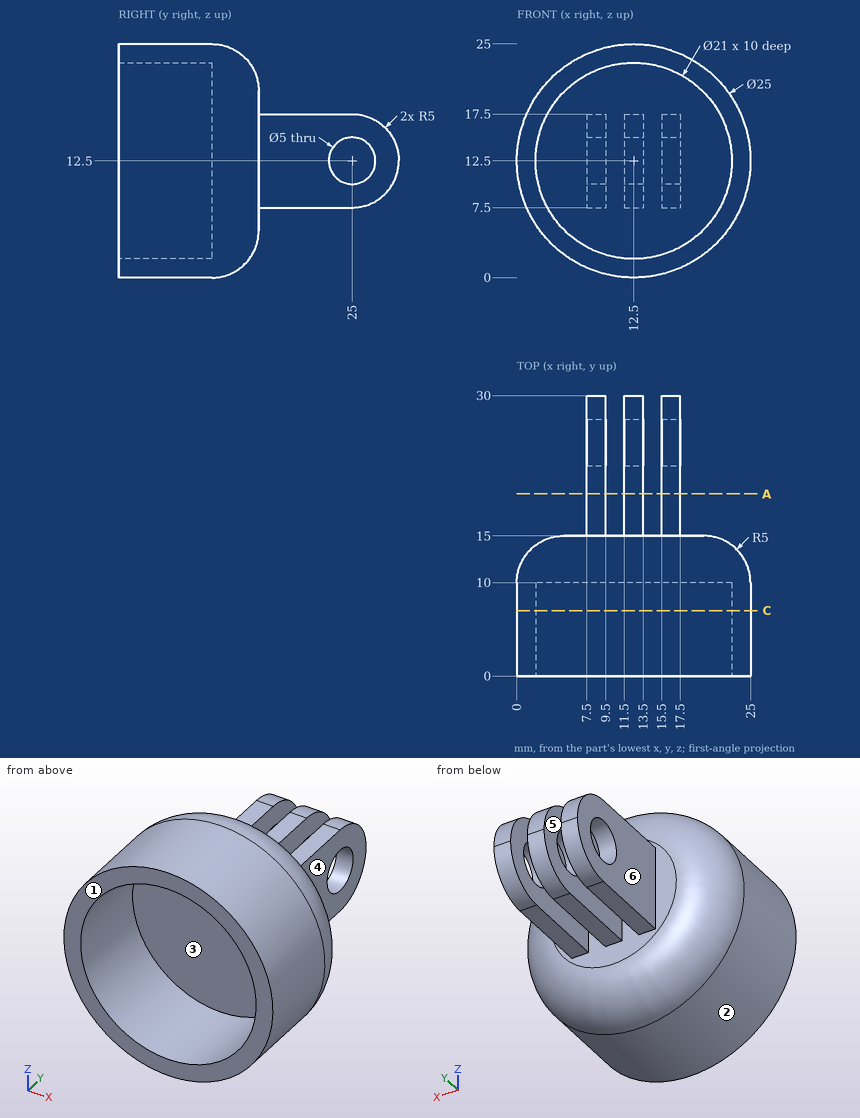
For this review, use the dimensioned drawing (mm, ordinates from the lowest corner) and the shaded views. A direction names the side the tool comes from. Round coordinates to 2 decimals unless told otherwise and drop trailing zeros. Order: outer loops, then holes, each group sorted by start corner. A loop starts at its lowest first (then second) coordinate and runs counter-clockwise, first axis right, second up.
1) Machinability: for the marked faces 4, 5 and 6, which of the approach directions +Z, -Z, +X, -X, +Y, -Y give a long, thin tool a straight path to every point of the face, cutting with its end or side? Answer none if there is none.
The answers:
face 4: +Z, -Z, +X, +Y
face 5: +Z, -Z, +Y
face 6: +Z, -Z, -X, +Y
2) For L1, parallel to Y at x = 12.9, z = 12.5; L2, parallel to X at y = 17, z = 14; L3, parallel to X at y = 7.75, z = 12.5, list the stretches that pass through material, from the lowest coordinate up.
The answers:
L1: y = 10 to 22.5, 27.5 to 30
L2: x = 7.5 to 9.5, 11.5 to 13.5, 15.5 to 17.5
L3: x = 0 to 2, 23 to 25
3) Clearance check with flat-ended pins moving along their axes: pin 1 Ø2 at (x, y) = (13, 18) entering from -Z; pin 2 Ø3 at (x, y) = (16, 12) entering from -Z; pin 3 Ø3 at (y, z) = (22, 12.5) entering from -X; pin 4 Ø12 at (x, z) = (18.5, 4) entering from -Y. State where each tip first meets the part, or that it passes through.
The answers:
pin 1: stops at z = 7.5
pin 2: stops at z = 0.33
pin 3: stops at x = 7.5
pin 4: stops at y = 0
4) Consider section A-A (y = 19.5). State the section outline as (x, z) points.
The answers:
outline: (7.5, 7.5) - (9.5, 7.5) - (9.5, 17.5) - (7.5, 17.5) - close; (11.5, 7.5) - (13.5, 7.5) - (13.5, 17.5) - (11.5, 17.5) - close; (15.5, 7.5) - (17.5, 7.5) - (17.5, 17.5) - (15.5, 17.5) - close
5) Consider section C-C (y = 7). State the section outline as (x, z) points.
The answers:
outline: circle Ø25 at (12.5, 12.5); hole circle Ø21 at (12.5, 12.5)
6) Draft analysis for pull direction X (two halves, no side actions). For the marked faces 1, 2 and 3, state which applies: released by +X, released by -X, zero draft, split by the parting line, or undercut.
The answers:
face 1: zero draft
face 2: split by the parting line
face 3: undercut
